from build123d import *

# Parameters (mm, degrees)
SKETCH_1_W                  = 88
SKETCH_1_H                  = 338
EXTRUDE_1_DEPTH             = 87
SKETCH_2_R                  = 2.5
CUT_EXTRUDE_1_DEPTH         = 196.105099882
PATTERN_LINEAR_1_COUNT      = 2
PATTERN_LINEAR_1_PITCH      = 100
PATTERN_LINEAR_1_COUNT_DIR2 = 2
PATTERN_LINEAR_1_PITCH_DIR2 = 62
SKETCH_3_R                  = 16.524250602
CUT_EXTRUDE_2_DEPTH         = 10


with BuildPart() as part:
    # 草图1 → 凸台-拉伸1 (new body)
    with BuildSketch(Plane(origin=(0, 0, 0), x_dir=(1, 0, 0), z_dir=(0, 1, 0))):
        Rectangle(SKETCH_1_W, SKETCH_1_H)
    extrude(amount=EXTRUDE_1_DEPTH)

    # 草图2 → 切除-拉伸1 (cut, through all)
    with BuildSketch(Plane.XZ):
        with Locations(Location((31, 114, 0), (0, 0, 270))):
            Circle(SKETCH_2_R)
    cut_extrude_1 = extrude(amount=-CUT_EXTRUDE_1_DEPTH, mode=Mode.SUBTRACT)

    # 阵列(线性)1: Cut-Extrude 1 2 × 2
    with Locations(*[(-j * PATTERN_LINEAR_1_PITCH_DIR2, 0, -i * PATTERN_LINEAR_1_PITCH) for i in range(PATTERN_LINEAR_1_COUNT) for j in range(PATTERN_LINEAR_1_COUNT_DIR2) if (i, j) != (0, 0)]):
        add(cut_extrude_1, mode=Mode.SUBTRACT)

    # 草图3 → 切除-拉伸2 (cut)
    with BuildSketch(Plane(origin=(0, 87, 0), x_dir=(1, 0, 0), z_dir=(0, 1, 0))):
        with Locations(Location((0, 96, 0), (0, 0, 270))):
            Circle(SKETCH_3_R)
    extrude(amount=-CUT_EXTRUDE_2_DEPTH, mode=Mode.SUBTRACT)


solid = part.part
For this review, take the finished solid that the model builds, in its own axes (mm). A direction names the side the tool comes from. Coordinates: 2 decimals unless noted, no trailing zeros. Order: outer loops, then holes, each group sorted by start corner. A loop starts at its lowest first (then second) coordinate and runs counter-clockwise, first axis right, second up. Notation, with made-up numbers: (84, 18) -> (109, 18) arc R26 cw to (109, 44) -> close; hole circle Ø7 at (-1, 59). An arc over 180 degrees is marked (long way). Return JSON: item names as keys, results as strings.
1. For line 1 (X direction, y = 42, z = 14); line 2 (Z direction, x = 1.5, y = 81); line 3 (X direction, y = 84.75, z = -96), list the stretches that pass through material, from the lowest coordinate up. Write a range as from..to.
Answer block:
{"line 1": "-44..-33.5, -28.5..28.5, 33.5..44", "line 2": "-169..-112.46, -79.54..169", "line 3": "-44..-16.52, 16.52..44"}
2. Machinability: for faces 1 (the flat face through (0, 77, -96)), 2 (the flat face through (-1, 87, -2)), which of the approach directions +Z, -Z, +X, -X, +Y, -Y give a long, thin tool a straight path to every point of the face, cutting with its end or side? Answer none if there is none.
Answer block:
{"face 1": "+Y", "face 2": "+Z, -Z, +X, -X, +Y"}
3. We need section A-A on z = -96. Write out the cut boundary in (x, y), and give its area (3 significant figures).
Answer block:
{"outline": "(-44, 0) -> (44, 0) -> (44, 87) -> (16.52, 87) -> (16.52, 77) -> (-16.52, 77) -> (-16.52, 87) -> (-44, 87) -> close", "area": "7,330 mm²"}
4. The part is to be moulded in two halves that separate along X. For faces 3 (the cylindrical face through (4.963, 82.07, -80.239)), 4 (the flat face through (-44, 43, 2)), 5 (the flat face through (-1, 0, -2)), say which applies: +X half, -X half, draft (parallel to the pull), parting line (faces both ways), or undercut.
Answer block:
{"face 3": "undercut", "face 4": "-X half", "face 5": "draft"}
